Source: three-view drawing plus pictorial views. Frame: mm from the lowest corner of the part. Give positions to 0.01 mm unless a question says otherwise; leave off trailing zeros. Order: outer loops, then holes, each group sorted by start corner. A loop starts at its lowest first (then second) coordinate and runs counter-clockwise, first axis right, second up. Notation, with made-up numbers: M 27.5,-17 L 39.5,-17 A20 cw 39.5,17 Z; hole C 4,2 d2. An arc over 180 degrees is marked long. Use CSV: the item, a comma, the result in double quotes. Start each with the question number.
Item 1: Ray query, probe 1 along X at (y, z) = (9, 2.9); probe 2 along Y at (x, z) = (74.5, 3.7); probe 3 along X at (y, z) = (28.5, 3.1). Return the intervals inside material, ascending. Write a range as from..to.
Item 2: Section query A-A on y = 13. Return loops of the section in (x, z), and give its area (3 significant figures).
Item 3: Section query C-C on z = 1.05. Count the separate pieces of the cut face and the enclosed holes in it, and give its area (3 significant figures).
Item 4: Section query B-B on x = 73.65. Return loops of the section in (y, z), and give its area (3 significant figures).
Item 5: Section query D-D on x = 39. Return loops of the section in (y, z), and give its area (3 significant figures).
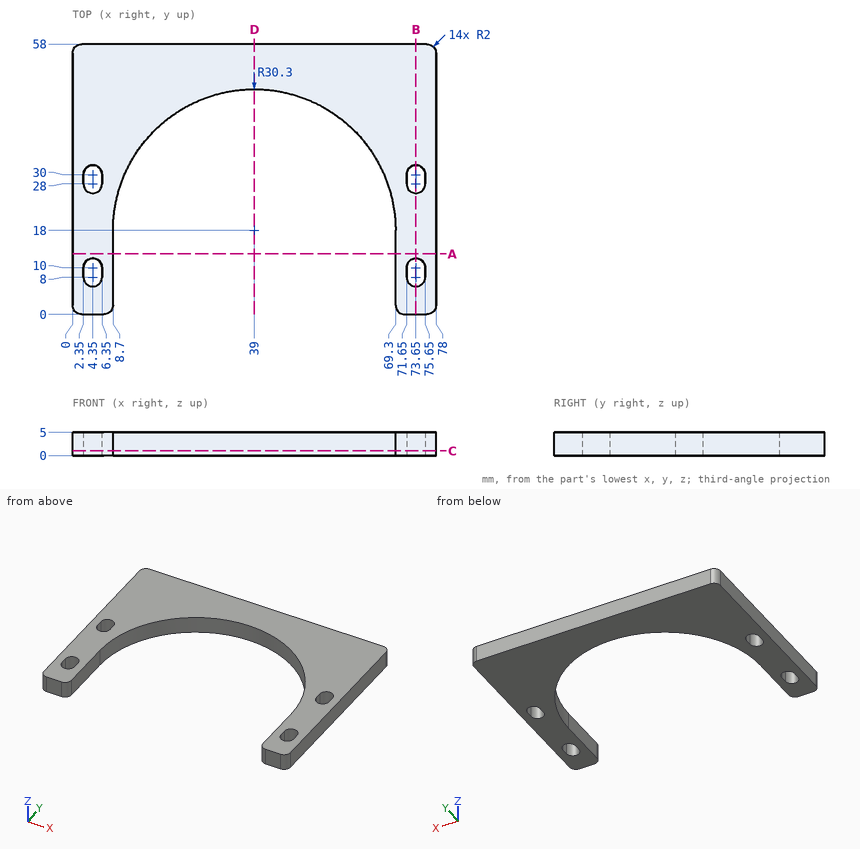
Verdict:
1,probe 1,"0..2.35, 6.35..8.7, 69.3..71.65, 75.65..78"
1,probe 2,"0..6.19, 11.81..26.19, 31.81..58"
1,probe 3,"0..2.35, 6.35..10.58, 67.42..71.65, 75.65..78"
2,outline,"M 0,0 L 8.7,0 L 8.7,5 L 0,5 Z; M 69.3,0 L 78,0 L 78,5 L 69.3,5 Z"
2,area,"87.0 mm2"
3,separate pieces,"1"
3,enclosed holes,"4"
3,area,"1,900 mm2"
4,outline,"M 0,0 L 6,0 L 6,5 L 0,5 Z; M 12,0 L 26,0 L 26,5 L 12,5 Z; M 32,0 L 58,0 L 58,5 L 32,5 Z"
4,area,"230 mm2"
5,outline,"M 48.3,0 L 58,0 L 58,5 L 48.3,5 Z"
5,area,"48.5 mm2"
